Read the model definition and answer for the solid it produces. Units are mm, in the model's axes. A direction names the side the tool comes from. Coordinates: 2 decimals unless noted, no trailing zeros. Loops run counter-clockwise (first coordinate to the right, second up) from the corner with the lowest first, then second, coordinate; pieces in that order, holes last. Notation, with made-up numbers: M 46,-26.75 L 100,-26.75 A25 ccw 100,5.25 Z; hole C 19,32.25 d3. An arc over 180 degrees is marked long. Use one line per item in the form item = value. Start each with the question number.
1. The part is cut by section A-A (x = 34.5). Give the vertices of the cut face in (y, z), plus the area to 3 significant figures.
2. Flat-ended cylindrical pins translate along their axes: pin 1 (10 mm diameter, centred on x = -42.5, z = -90, fed in from -Y); pin 2 (1 mm diameter, centred on x = -1, y = 1.5, fed in from +Z); pin 3 (1.6 mm diameter, centred on y = 2, z = -181, fed in from +X); pin 4 (3.5 mm diameter, centred on x = -175.5, y = 2.5, fed in from -Z). Find the tip coordinate at first contact, or state that the pin passes through.
3. Find the intervals of material crossed by probe 1 along Z at (x, y) = (5, 6); probe 2 along X at (y, z) = (4, 60); probe 3 along Z at (x, y) = (-89.5, 1.5), in increasing order. Write a range as [from, to].
4. For a pull along Z with two mould halves and no side action, classify faces 3 (the cylindrical face through (-114.85, 3.22, -49.68)), 4 (the flat face through (-2, 6.35, 120)), 5 (the cylindrical face through (150.48, 3.22, -93.24)), 6 (the cylindrical face through (-174.18, 3.22, -180.33)) as released by +Z, released by -Z, zero draft, split by the parting line, or undercut.
5. A tool of negligible diameter and unlimited length cuts with its end or side. For faces 1 (the cylindrical face through (174.18, 3.22, -180.33)), 2 (the cylindrical face through (-150.33, 3.22, -93.39)), from which of +Z, -Z, +X, -X, +Y, -Y can it reach the whole face along a straight path? Write none if from no direction.
6. The part is cut by section B-B (y = 3.5). Give the number of separate pieces and of enclosed holes in the cut face, plus the area to 3 significant figures.
from build123d import *

# Parameters (mm, degrees)
SKETCH2_W               = 355.6
SKETCH2_H               = 368.3
BOSS_EXTRUDE1_DEPTH     = 6.35
FILLET1_R               = 12.7
MOUNTING_HOLES_DEPTH    = 7.35
PLUNGER_CUTOUT_DEPTH    = 7.35
F_1_4_20_TAPPED_HOLE2_D = 5.1054
CENTERING_MARKERS_DEPTH = 7.35
FILLET2_R               = 1.5875
F_1_4_20_TAPPED_HOLE5_D = 5.1054
SKETCH17_R              = 3.571875
CUT_EXTRUDE1_DEPTH      = 7.35


with BuildPart() as part:
    # Sketch2 → Boss-Extrude1 (new body)
    with BuildSketch(Plane(origin=(0, 0, 0), x_dir=(1, 0, 0), z_dir=(0, 1, 0))):
        Rectangle(SKETCH2_W, SKETCH2_H)
    extrude(amount=BOSS_EXTRUDE1_DEPTH)

    # Fillet1
    fillet1_edges = [part.edges().sort_by_distance(p)[0] for p in [
        (177.8, 3.175, 184.15),
        (-177.8, 3.175, 184.15),
        (-177.8, 3.175, -184.15),
        (177.8, 3.175, -184.15),
    ]]
    fillet(fillet1_edges, radius=FILLET1_R)

    # Sketch3 → MOUNTING HOLES (cut, through all)
    with BuildSketch(Plane(origin=(0, 6.35, 0), x_dir=(1, 0, 0), z_dir=(0, 1, 0))):
        with BuildLine():
            Line((-88.10625, 174.228125), (-78.58125, 174.228125))
            ThreePointArc((-78.58125, 174.228125), (-74.215625, 169.8625), (-78.58125, 165.496875))
            Line((-78.58125, 165.496875), (-88.10625, 165.496875))
            ThreePointArc((-88.10625, 165.496875), (-92.471875, 169.8625), (-88.10625, 174.228125))
        make_face()
        with BuildLine():
            Line((88.10625, 165.496875), (78.58125, 165.496875))
            ThreePointArc((78.58125, 165.496875), (74.215625, 169.8625), (78.58125, 174.228125))
            Line((78.58125, 174.228125), (88.10625, 174.228125))
            ThreePointArc((88.10625, 174.228125), (92.471875, 169.8625), (88.10625, 165.496875))
        make_face()
        with BuildLine():
            Line((-88.10625, -165.496875), (-78.58125, -165.496875))
            ThreePointArc((-78.58125, -165.496875), (-74.215625, -169.8625), (-78.58125, -174.228125))
            Line((-78.58125, -174.228125), (-88.10625, -174.228125))
            ThreePointArc((-88.10625, -174.228125), (-92.471875, -169.8625), (-88.10625, -165.496875))
        make_face()
        with BuildLine():
            Line((78.58125, -165.496875), (88.10625, -165.496875))
            ThreePointArc((88.10625, -165.496875), (92.471875, -169.8625), (88.10625, -174.228125))
            Line((88.10625, -174.228125), (78.58125, -174.228125))
            ThreePointArc((78.58125, -174.228125), (74.215625, -169.8625), (78.58125, -165.496875))
        make_face()
    extrude(amount=-MOUNTING_HOLES_DEPTH, mode=Mode.SUBTRACT)

    # Sketch4 → PLUNGER CUTOUT (cut, through all)
    with BuildSketch(Plane(origin=(0, 6.35, 0), x_dir=(1, 0, 0), z_dir=(0, 1, 0))):
        with BuildLine():
            Line((-99.28098, -96.10598), (99.28098, -96.10598))
            ThreePointArc((99.28098, -96.10598), (108.261236121, -92.386236121), (111.98098, -83.40598))
            Line((111.98098, -83.40598), (111.98098, 42.86885))
            ThreePointArc((111.98098, 42.86885), (114.770787909, 49.604042091), (121.50598, 52.39385))
            Line((121.50598, 52.39385), (143.66875, 52.39385))
            ThreePointArc((143.66875, 52.39385), (150.403942091, 55.183657909), (153.19375, 61.91885))
            Line((153.19375, 61.91885), (153.19375, 86.58098))
            ThreePointArc((153.19375, 86.58098), (150.403942091, 93.316172091), (143.66875, 96.10598))
            Line((143.66875, 96.10598), (-143.66875, 96.10598))
            ThreePointArc((-143.66875, 96.10598), (-150.403942091, 93.316172091), (-153.19375, 86.58098))
            Line((-153.19375, 86.58098), (-153.19375, 61.91885))
            ThreePointArc((-153.19375, 61.91885), (-150.403942091, 55.183657909), (-143.66875, 52.39385))
            Line((-143.66875, 52.39385), (-121.50598, 52.39385))
            ThreePointArc((-121.50598, 52.39385), (-114.770787909, 49.604042091), (-111.98098, 42.86885))
            Line((-111.98098, 42.86885), (-111.98098, -83.40598))
            ThreePointArc((-111.98098, -83.40598), (-108.261236121, -92.386236121), (-99.28098, -96.10598))
        make_face()
    extrude(amount=-PLUNGER_CUTOUT_DEPTH, mode=Mode.SUBTRACT)

    # 1/4-20 Tapped Hole2 (through all)
    with Locations(Plane(origin=(0, 6.35, 0), x_dir=(1, 0, 0), z_dir=(0, 1, 0))):
        with Locations((-80.16748, -108.81868), (-48.41748, -108.81868), (48.41748, -108.81868), (80.16748, -108.81868), (80.16748, 108.81868), (48.41748, 108.81868), (-48.41748, 108.81868), (-80.16748, 108.81868)):
            Hole(F_1_4_20_TAPPED_HOLE2_D / 2)

    # Sketch10 → CENTERING MARKERS (cut, through all)
    with BuildSketch(Plane(origin=(0, 6.35, 0), x_dir=(1, 0, 0), z_dir=(0, 1, 0))):
        with BuildLine():
            Line((-0.79375, -179.3875), (-0.79375, -184.15))
            Line((-0.79375, -184.15), (0.79375, -184.15))
            Line((0.79375, -184.15), (0.79375, -179.3875))
            ThreePointArc((0.79375, -179.3875), (0, -178.59375), (-0.79375, -179.3875))
        make_face()
        with BuildLine():
            Line((-173.0375, 0.79375), (-177.8, 0.79375))
            Line((-177.8, 0.79375), (-177.8, -0.79375))
            Line((-177.8, -0.79375), (-173.0375, -0.79375))
            ThreePointArc((-173.0375, -0.79375), (-172.24375, 0), (-173.0375, 0.79375))
        make_face()
        with BuildLine():
            Line((173.0375, 0.79375), (177.8, 0.79375))
            Line((177.8, 0.79375), (177.8, -0.79375))
            Line((177.8, -0.79375), (173.0375, -0.79375))
            ThreePointArc((173.0375, -0.79375), (172.24375, 0), (173.0375, 0.79375))
        make_face()
        with BuildLine():
            Line((-0.79375, 179.3875), (-0.79375, 184.15))
            Line((-0.79375, 184.15), (0.79375, 184.15))
            Line((0.79375, 184.15), (0.79375, 179.3875))
            ThreePointArc((0.79375, 179.3875), (0, 178.59375), (-0.79375, 179.3875))
        make_face()
    extrude(amount=-CENTERING_MARKERS_DEPTH, mode=Mode.SUBTRACT)

    # Fillet2
    fillet2_edges = [part.edges().sort_by_distance(p)[0] for p in [
        (177.8, 3.175, -0.79375),
        (177.8, 3.175, 0.79375),
        (0.79375, 3.175, 184.15),
        (-0.79375, 3.175, 184.15),
        (-0.79375, 3.175, -184.15),
        (0.79375, 3.175, -184.15),
        (-177.8, 3.175, 0.79375),
        (-177.8, 3.175, -0.79375),
    ]]
    fillet(fillet2_edges, radius=FILLET2_R)

    # 1/4-20 Tapped Hole5 (through all)
    with Locations(Plane(origin=(0, 6.35, 0), x_dir=(1, 0, 0), z_dir=(0, 1, 0))):
        with Locations((-144.526, -17.4752), (-144.526, -80.9752), (-118.33225, -39.6875), (-118.33225, 39.6875), (118.33225, 39.6875), (118.33225, -39.6875), (144.526, -17.4752), (144.526, -80.9752)):
            Hole(F_1_4_20_TAPPED_HOLE5_D / 2)

    # Sketch17 → Cut-Extrude1 (cut, through all)
    with BuildSketch(Plane(origin=(0, 6.35, 0), x_dir=(1, 0, 0), z_dir=(0, 1, 0))):
        with Locations((-138.96975, 36.5125)):
            Circle(SKETCH17_R)
        with Locations((-138.96975, 14.2875)):
            Circle(SKETCH17_R)
        with Locations((138.96975, 14.2875)):
            Circle(SKETCH17_R)
        with Locations((138.96975, 36.5125)):
            Circle(SKETCH17_R)
    extrude(amount=-CUT_EXTRUDE1_DEPTH, mode=Mode.SUBTRACT)


solid = part.part
Computed values:
q1.outline = M 0,-184.15 L 6.35,-184.15 L 6.35,-96.11 L 0,-96.11 Z; M 0,96.11 L 6.35,96.11 L 6.35,184.15 L 0,184.15 Z
q1.area = 1,120 mm²
q2.pin_1 = through
q2.pin_2 = 183.88
q2.pin_3 = 174.3
q2.pin_4 = -180.75
q3.probe_1 = [-184.15, -96.11], [96.11, 184.15]
q3.probe_2 = [-177.8, -111.98], [111.98, 177.8]
q3.probe_3 = [-184.15, -174], [-165.73, -96.11], [96.11, 165.73], [174, 184.15]
q4.face_3 = undercut
q4.face_4 = zero draft
q4.face_5 = undercut
q4.face_6 = released by -Z
q5.face_1 = -Z, +X, +Y, -Y
q5.face_2 = +Y, -Y
q6.separate_pieces = 1
q6.enclosed_holes = 25
q6.area = 83,200 mm²
